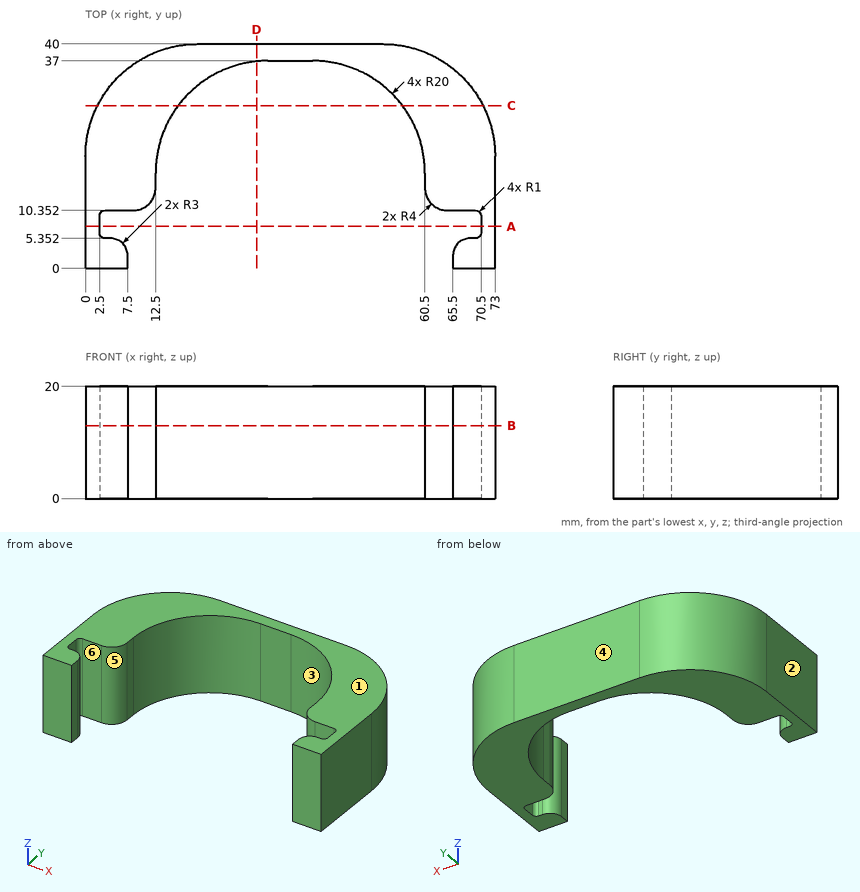
Study the drawing (mm; zero at the part's minimum x, y, z) and answer. A direction names the side the tool comes from. Coordinates: 2 decimals unless noted, no trailing zeros. Write each loop counter-clockwise with the first axis right and the second up, starting at its lowest first coordinate (ties: lowest second). Pieces come first, ordered by that corner, then holes. Notation, with made-up numbers: M -26,-14.5 L -12,-14.5 A19 cw -12,-9.5 Z; hole C -22,-6.75 d1. An arc over 180 degrees is marked long. Use a Markdown table: item, result. Add a question column.
1. Section B-B (z = 13) is taken. Give the vertices of the cut face in (x, y).
2. Section A-A (y = 7.5) is taken. Give the vertices of the cut face in (x, z), plus the area to 3 significant figures.
3. Section C-C (y = 29) is taken. Give the vertices of the cut face in (x, z).
4. Straight lines are drawn through the part: line 1 along X through (y, z) = (8, 10.5); line 2 along Y through (x, z) = (39, 5.5); line 3 along X through (y, z) = (24, 10.75) (1 decimal). For each, find the intervals that lie inside material, in ascending order. Write a range as [from, to].
5. Given P1, Ø1.1, axis at x = 4, z = 13.5, coming from the +Y side; P2, Ø6, axis at y = 23.5, z = 14.5, coming from the +X side; P3, Ø9, axis at x = 36.5, z = 14, coming from the -Y side, each flat-ended and moving along its own axis, determine where each tip first touches the part or whether it passes through.
6. Section D-D (x = 30.5) is taken. Give the vertices of the cut face in (y, z), plus the area to 3 significant figures.
7. Which of the six approach directions +Z, -Z, +X, -X, +Y, -Y give full straight-line access (tool end or side, diameter ignored) to the marked faces 4, 5 and 6?
8. For a pull along X with two mould halves and no side action, classify the marked faces 1, 2 and 3 as +X half, -X half, draft (parallel to the pull), parting line (faces both ways), or undercut.
Data:
| question | item | result |
|---|---|---|
| 1 | outline | M 0,0 L 7.5,0 L 7.5,2.35 A3 ccw 4.5,5.35 L 3.5,5.35 A1 cw 2.5,6.35 L 2.5,9.35 A1 cw 3.5,10.35 L 8.5,10.35 A4 ccw 12.5,14.35 L 12.5,17 A20 cw 32.5,37 L 40.5,37 A20 cw 60.5,17 L 60.5,14.35 A4 ccw 64.5,10.35 L 69.5,10.35 A1 cw 70.5,9.35 L 70.5,6.35 A1 cw 69.5,5.35 L 68.5,5.35 A3 ccw 65.5,2.35 L 65.5,0 L 73,0 L 73,20 A20 ccw 53,40 L 20,40 A20 ccw 0,20 Z |
| 2 | outline | M 0,0 L 2.5,0 L 2.5,20 L 0,20 Z; M 70.5,0 L 73,0 L 73,20 L 70.5,20 Z |
| 2 | area | 100 mm2 |
| 3 | outline | M 2.14,0 L 16.5,0 L 16.5,20 L 2.14,20 Z; M 56.5,0 L 70.86,0 L 70.86,20 L 56.5,20 Z |
| 4 | line 1 | x = [0, 2.5], [70.5, 73] |
| 4 | line 2 | y = [37, 40] |
| 4 | line 3 | x = [0.4, 13.8], [59.2, 72.6] |
| 5 | P1 | stops at y = 32.7 |
| 5 | P2 | stops at x = 72.99 |
| 5 | P3 | stops at y = 36.99 |
| 6 | outline | M 36.9,0 L 40,0 L 40,20 L 36.9,20 Z |
| 6 | area | 62.0 mm2 |
| 7 | face 4 | +Z, -Z, +X, -X, +Y |
| 7 | face 5 | +Z, -Z, -Y |
| 7 | face 6 | +Z, -Z |
| 8 | face 1 | draft |
| 8 | face 2 | -X half |
| 8 | face 3 | undercut |
